The model under review builds one solid part; all positions refer to its coordinate system, in mm. A direction names the side the tool comes from. Coordinates: 2 decimals unless noted, no trailing zeros. Write each loop counter-clockwise with the first axis right and the second up, starting at its lowest first coordinate (ties: lowest second). Pieces come first, ordered by that corner, then holes. Notation, with made-up numbers: M 81.25,-1.75 L 115.25,-1.75 A21 ccw 115.25,7.25 Z; hole C 79.5,63.25 d10. An arc over 180 degrees is marked long. Answer as a JSON object with one key per item and string values.
```python
from build123d import *

# Parameters (mm, degrees)
F0_W     = 30
F0_H     = 50
F0_R     = 5
F1_DEPTH = 2
F2_DEPTH = 2


with BuildPart() as f1:
    # F0 (on Top) → F1 (new body)
    with BuildSketch(Plane.XY):
        Rectangle(F0_W, F0_H)
        Circle(F0_R, mode=Mode.SUBTRACT)
        Circle(F0_R)
    extrude(amount=F1_DEPTH)

    # F0 (on Top) → F2 (join)
    with BuildSketch(Plane.XY):
        Circle(F0_R)
    extrude(amount=-F2_DEPTH)


solid = f1.part
```
(1) Add section B-B on x = 0. Give the boundary of the cut face in (y, z), and give its area (3 significant figures).
Results list:
{"outline": "M -25,0 L -5,0 L -5,-2 L 5,-2 L 5,0 L 25,0 L 25,2 L -25,2 Z", "area": "120 mm²"}
(2) For faces 1 (the face through (-1.08, -4.88, -0.99)), 2 (the face through (0, -25, 1)), list the 3-axis set-ups (+Z, -Z, +X, -X, +Y, -Y) from which the entire face can be reached by the end or side of a thin tool; tool diameter is ignored.
Results list:
{"face 1": "-Z", "face 2": "+Z, -Z, +X, -X, -Y"}
(3) Add section D-D on x = -11.5. Give the boundary of the cut face in (y, z).
Results list:
{"outline": "M -25,0 L 25,0 L 25,2 L -25,2 Z"}
(4) Add section C-C on z = -1.45. Give the boundary of the cut face in (x, y), and give its area (3 significant figures).
Results list:
{"outline": "C 0,0 d10", "area": "78.5 mm²"}
(5) For pin 1 Ø2 at (y, z) = (-2, -0.5) entering from +X; pin 2 Ø3 at (x, y) = (6.5, 3) entering from -Z, all flat-tipped, find the tip position at first contact; note any pin that passes through.
Results list:
{"pin 1": "x = 15", "pin 2": "z = 0"}
(6) Wall thickness on line 1 along Z through (x, y) = (-6.5, -20.5); line 2 along Y through (x, z) = (2, -1.55): over which ranges is each line inside the solid? List them lowest first. Write a range as from..to.
Results list:
{"line 1": "0..2", "line 2": "-4.58..4.58"}
(7) Add section A-A on y = 3. Give the boundary of the cut face in (x, z), and give its area (3 significant figures).
Results list:
{"outline": "M -15,0 L -4,0 L -4,-2 L 4,-2 L 4,0 L 15,0 L 15,2 L -15,2 Z", "area": "76.0 mm²"}
